Geometry check sheet. Reference: the model listing, model coordinates, mm. A direction names the side the tool comes from. Coordinates: 2 decimals unless noted, no trailing zeros. Answer as a JSON object with one key per item and string values. Group by question number.
```python
from build123d import *

# Parameters (mm, degrees)
SKETCH1_R          = 3.4036
EXTRUDE1_DEPTH     = 215.9
CUT_EXTRUDE1_DEPTH = 436.22027791
CUT_EXTRUDE2_DEPTH = 3.048
CUT_EXTRUDE5_REACH = 437.22
CUT_EXTRUDE6_DEPTH = 3.048


with BuildPart() as part:
    # Sketch1 → Extrude1 (new, symmetric)
    with BuildSketch(Plane.XY):
        with BuildLine():
            Line((-20, 16.952), (-20, 4.7625))
            ThreePointArc((-20, 4.7625), (-19.776815367, 4.223684633), (-19.238, 4.0005))
            Line((-19.238, 4.0005), (-16.2662, 4.0005))
            ThreePointArc((-16.2662, 4.0005), (-15.727384633, 4.223684633), (-15.5042, 4.7625))
            Line((-15.5042, 4.7625), (-15.5042, 10.485558599))
            ThreePointArc((-15.5042, 10.485558599), (-15.033804775, 11.189554802), (-14.203384633, 11.024373966))
            Line((-14.203384633, 11.024373966), (-8.635059555, 5.456048889))
            ThreePointArc((-8.635059555, 5.456048889), (-7.985348265, 4.483687227), (-7.7572, 3.336708444))
            Line((-7.7572, 3.336708444), (-7.7572, -3.336708444))
            ThreePointArc((-7.7572, -3.336708444), (-7.985348265, -4.483687227), (-8.635059555, -5.456048889))
            Line((-8.635059555, -5.456048889), (-14.203384633, -11.024373966))
            ThreePointArc((-14.203384633, -11.024373966), (-15.033804775, -11.189554802), (-15.5042, -10.485558599))
            Line((-15.5042, -10.485558599), (-15.5042, -4.7625))
            ThreePointArc((-15.5042, -4.7625), (-15.727384633, -4.223684633), (-16.2662, -4.0005))
            Line((-16.2662, -4.0005), (-19.238, -4.0005))
            ThreePointArc((-19.238, -4.0005), (-19.776815367, -4.223684633), (-20, -4.7625))
            Line((-20, -4.7625), (-20, -16.952))
            ThreePointArc((-20, -16.952), (-19.107261469, -19.107261469), (-16.952, -20))
            Line((-16.952, -20), (-4.7625, -20))
            ThreePointArc((-4.7625, -20), (-4.223684633, -19.776815367), (-4.0005, -19.238))
            Line((-4.0005, -19.238), (-4.0005, -16.2662))
            ThreePointArc((-4.0005, -16.2662), (-4.223684633, -15.727384633), (-4.7625, -15.5042))
            Line((-4.7625, -15.5042), (-10.485558599, -15.5042))
            ThreePointArc((-10.485558599, -15.5042), (-11.189554802, -15.033804775), (-11.024373966, -14.203384633))
            Line((-11.024373966, -14.203384633), (-5.456048889, -8.635059555))
            ThreePointArc((-5.456048889, -8.635059555), (-4.483687227, -7.985348265), (-3.336708444, -7.7572))
            Line((-3.336708444, -7.7572), (3.336708444, -7.7572))
            ThreePointArc((3.336708444, -7.7572), (4.483687227, -7.985348265), (5.456048889, -8.635059555))
            Line((5.456048889, -8.635059555), (11.024373966, -14.203384633))
            ThreePointArc((11.024373966, -14.203384633), (11.189554802, -15.033804775), (10.485558599, -15.5042))
            Line((10.485558599, -15.5042), (4.7625, -15.5042))
            ThreePointArc((4.7625, -15.5042), (4.223684633, -15.727384633), (4.0005, -16.2662))
            Line((4.0005, -16.2662), (4.0005, -19.238))
            ThreePointArc((4.0005, -19.238), (4.223684633, -19.776815367), (4.7625, -20))
            Line((4.7625, -20), (16.952, -20))
            ThreePointArc((16.952, -20), (19.107261469, -19.107261469), (20, -16.952))
            Line((20, -16.952), (20, -4.7625))
            ThreePointArc((20, -4.7625), (19.776815367, -4.223684633), (19.238, -4.0005))
            Line((19.238, -4.0005), (16.2662, -4.0005))
            ThreePointArc((16.2662, -4.0005), (15.727384633, -4.223684633), (15.5042, -4.7625))
            Line((15.5042, -4.7625), (15.5042, -10.485558599))
            ThreePointArc((15.5042, -10.485558599), (15.033804775, -11.189554802), (14.203384633, -11.024373966))
            Line((14.203384633, -11.024373966), (8.635059555, -5.456048889))
            ThreePointArc((8.635059555, -5.456048889), (7.985348265, -4.483687227), (7.7572, -3.336708444))
            Line((7.7572, -3.336708444), (7.7572, 3.336708444))
            ThreePointArc((7.7572, 3.336708444), (7.985348265, 4.483687227), (8.635059555, 5.456048889))
            Line((8.635059555, 5.456048889), (14.203384633, 11.024373966))
            ThreePointArc((14.203384633, 11.024373966), (15.033804775, 11.189554802), (15.5042, 10.485558599))
            Line((15.5042, 10.485558599), (15.5042, 4.7625))
            ThreePointArc((15.5042, 4.7625), (15.727384633, 4.223684633), (16.2662, 4.0005))
            Line((16.2662, 4.0005), (19.238, 4.0005))
            ThreePointArc((19.238, 4.0005), (19.776815367, 4.223684633), (20, 4.7625))
            Line((20, 4.7625), (20, 16.952))
            ThreePointArc((20, 16.952), (19.107261469, 19.107261469), (16.952, 20))
            Line((16.952, 20), (4.7625, 20))
            ThreePointArc((4.7625, 20), (4.223684633, 19.776815367), (4.0005, 19.238))
            Line((4.0005, 19.238), (4.0005, 16.2662))
            ThreePointArc((4.0005, 16.2662), (4.223684633, 15.727384633), (4.7625, 15.5042))
            Line((4.7625, 15.5042), (10.485558599, 15.5042))
            ThreePointArc((10.485558599, 15.5042), (11.189554802, 15.033804775), (11.024373966, 14.203384633))
            Line((11.024373966, 14.203384633), (5.456048889, 8.635059555))
            ThreePointArc((5.456048889, 8.635059555), (4.483687227, 7.985348265), (3.336708444, 7.7572))
            Line((3.336708444, 7.7572), (-3.336708444, 7.7572))
            ThreePointArc((-3.336708444, 7.7572), (-4.483687227, 7.985348265), (-5.456048889, 8.635059555))
            Line((-5.456048889, 8.635059555), (-11.024373966, 14.203384633))
            ThreePointArc((-11.024373966, 14.203384633), (-11.189554802, 15.033804775), (-10.485558599, 15.5042))
            Line((-10.485558599, 15.5042), (-4.7625, 15.5042))
            ThreePointArc((-4.7625, 15.5042), (-4.223684633, 15.727384633), (-4.0005, 16.2662))
            Line((-4.0005, 16.2662), (-4.0005, 19.238))
            ThreePointArc((-4.0005, 19.238), (-4.223684633, 19.776815367), (-4.7625, 20))
            Line((-4.7625, 20), (-16.952, 20))
            ThreePointArc((-16.952, 20), (-19.107261469, 19.107261469), (-20, 16.952))
        make_face()
        Circle(SKETCH1_R, mode=Mode.SUBTRACT)
    extrude(amount=EXTRUDE1_DEPTH, both=True)

    # Sketch3 → Cut-Extrude1 (cut, through all)
    with BuildSketch(Plane(origin=(-16.952, 20, 215.9), x_dir=(0, 0, 1), z_dir=(-1, 0, 0))):
        Polygon((0, 0), (-40, -40), (0, -40), align=None)
    extrude(amount=-CUT_EXTRUDE1_DEPTH, mode=Mode.SUBTRACT)

    # Sketch4 → Cut-Extrude2 (cut)
    with BuildSketch(Plane(origin=(-16.952, 0, 0), x_dir=(0, 0, -1), z_dir=(1, 0, 0))):
        Polygon((-215.9, 20), (-215.9, -20), (-175.9, -20), align=None)
    extrude(amount=-CUT_EXTRUDE2_DEPTH, mode=Mode.SUBTRACT)

    # Cut-Extrude5: up to this face of the body (flat: up to its plane)
    cut_extrude5_end = Plane(part.part.faces().sort_by_distance((20, 10.886545588, -4.556727206))[0])
    # Sketch9 → Cut-Extrude5 (cut, up to the picked face)
    with BuildSketch(Plane(origin=(-16.952, 20, 215.9), x_dir=(0, 0, 1), z_dir=(-1, 0, 0)), mode=Mode.PRIVATE) as cut_extrude5_sk1:
        Polygon((-431.8, 0), (-391.8, -40), (-431.8, -40), align=None)
    cut_extrude5_tool1 = split(extrude(cut_extrude5_sk1.sketch, amount=-CUT_EXTRUDE5_REACH, mode=Mode.PRIVATE), bisect_by=cut_extrude5_end, keep=Keep.BOTH, mode=Mode.PRIVATE)
    add(cut_extrude5_tool1.solids().sort_by(Axis((-16.952, -6.666667, -202.566667), (1, 0, 0)))[0], mode=Mode.SUBTRACT)

    # Sketch11 → Cut-Extrude6 (cut)
    with BuildSketch(Plane(origin=(-16.952, 0, 0), x_dir=(0, 0, -1), z_dir=(1, 0, 0))):
        Polygon((175.9, -20), (215.9, 20), (215.9, -20), align=None)
    extrude(amount=-CUT_EXTRUDE6_DEPTH, mode=Mode.SUBTRACT)


solid = part.part
```
1) Draft check along X on faces 1 (the flat face through (0, -7.757, 3)), 2 (the cylindrical face through (3.144, -1.304, -2.791)), 3 (the flat face through (4.7, -0.3, -195.6)), 4 (the flat face through (-20, 11, 3)). Enter one of: +X half, -X half, draft (parallel to the pull), parting line (faces both ways), or undercut.
2) Set-up check for faces 5 (the flat face through (0, 7.757, 3)), 6 (the flat face through (7.757, 0, 3)), 7 (the flat face through (-7.757, 0, 3)), 8 (the flat face through (20, 11, 3)), 9 (the flat face through (-20, -11, 3)): record each of +Z, -Z, +X, -X, +Y, -Y from which the full face is reachable in a straight line by a thin tool's end or side.
3) Go/stop test with flat-tipped pins: pin 1 Ø6 at (x, y) = (3, 3) entering from +Z; pin 2 Ø0.9 at (y, z) = (-18, -18.5) entering from +X; pin 3 Ø3 at (x, y) = (2, 8) entering from +Z. Record where each tip stops, or that it passes through.
4) Material ranges on probe 1 along X at (y, z) = (14.5, 49.5); probe 2 along Y at (x, z) = (11, 165); probe 3 along X at (y, z) = (0, 43), recorded low to high. Write a range as [from, to].
Entries:
{
 "1": {"face 1": "undercut", "face 2": "undercut", "face 3": "draft", "face 4": "-X half"},
 "2": {"face 5": "+Z, -Z, +Y", "face 6": "+Z, -Z, +X", "face 7": "+Z, -Z, -X", "face 8": "+Z, -Z, +X, +Y, -Y", "face 9": "+Z, -Z, -X, +Y, -Y"},
 "3": {"pin 1": "z = 201.9", "pin 2": "x = 19.94", "pin 3": "z = 203.66"},
 "4": {"probe 1": "[-20, -11.21], [11.21, 20]", "probe 2": "[-20, -15.3], [-14.18, -7.82], [7.82, 14.18], [15.3, 20]", "probe 3": "[-7.76, -3.4], [3.4, 7.76]"}
}
